Read the model definition and answer for the solid it produces. Units are mm, in the model's axes. Give positions to 0.01 mm unless a question says otherwise; leave off trailing zeros. Loops run counter-clockwise (first coordinate to the right, second up) from the corner with the lowest first, then second, coordinate; pieces in that order, holes last. Notation, with made-up numbers: (-36.5, 9.5) - (2.5, 9.5) arc R19 cw to (2.5, 27.5) - close; hole circle Ø5 at (34.5, -31). An arc over 180 degrees is marked (long way). Put each result on its own line as item: value. Start each with the question number.
1. Given pin 1 Ø1.5 at (y, z) = (30.5, 11) entering from -X; pin 2 Ø6 at (x, z) = (14, 3) entering from -Y; pin 3 Ø5 at (x, z) = (-12, 9.5) entering from +Y; pin 4 Ø1.5 at (x, z) = (-0.5, 7) entering from +Y, each flat-ended and moving along its own axis, determine where each tip first touches the part or whether it passes through.
2. A cutting plane is placed at D-D, the plane x = 11. Determine the outline of the cut face in (y, z), plus the area to 3 significant figures.
3. Consider L1, parallel to X at y = 7, z = 8; L2, parallel to Y at x = 0, z = 4.5; L3, parallel to Y at x = 11, z = 10.5. Determine where each line is inside the solid, lowest interval first. Write a range as from..to.
4. A cutting plane is placed at B-B, the plane z = 13.25. Determine the outline of the cut face in (x, y), plus the area to 3 significant figures.
5. A cutting plane is placed at C-C, the plane y = 27.3. Determine the outline of the cut face in (x, z), plus the area to 3 significant figures.
6. For a pull along X with two mould halves and no side action, classify faces 1 (the cylindrical face through (10.46, 3.76, 7.99)), 2 (the cylindrical face through (-16.57, -16.8, 7.76)), 3 (the cylindrical face through (-0.54, 24.86, 7.99)), 4 (the flat face through (0, 9, 0)) as released by +X, released by -X, zero draft, split by the parting line, or undercut.
7. A cutting plane is placed at A-A, the plane y = 6.2. Determine the outline of the cut face in (x, z), plus the area to 4 significant figures.
```python
from build123d import *

# Parameters (mm, degrees)
F1_DEPTH = 15.75
F2_R     = 2.5
F3_DEPTH = 15.751


with BuildPart() as f1:
    # F0 (on Top) → F1 (new body)
    with BuildSketch(Plane.XY):
        with BuildLine():
            ThreePointArc((-18, -13.3), (-16.535534, -16.835534), (-13, -18.3))
            Line((-13, -18.3), (13, -18.3))
            ThreePointArc((13, -18.3), (16.535534, -16.835534), (18, -13.3))
            Line((18, -13.3), (18, 18.3))
            ThreePointArc((18, 18.3), (0, 36.3), (-18, 18.3))
            Line((-18, 18.3), (-18, -13.3))
        make_face()
    extrude(amount=F1_DEPTH)

    # F2 (on face) → F3 (cut, through all)
    with BuildSketch(Plane.XY.offset(15.75)):
        with Locations((0, 27.3)):
            Circle(F2_R)
        with Locations((-11, 6.2)):
            Circle(F2_R)
        with Locations((11, 6.2)):
            Circle(F2_R)
    extrude(amount=-F3_DEPTH, mode=Mode.SUBTRACT)


solid = f1.part
```
Return value:
1. pin 1: stops at x = -13.89
1. pin 2: stops at y = -18.3
1. pin 3: stops at y = 33.59
1. pin 4: stops at y = 36.3
2. outline: (-18.3, 0) - (3.7, 0) - (3.7, 15.75) - (-18.3, 15.75) - close; (8.7, 0) - (32.55, 0) - (32.55, 15.75) - (8.7, 15.75) - close
2. area: 722 mm2
3. L1: x = -18..-13.37, -8.63..8.63, 13.37..18
3. L2: y = -18.3..24.8, 29.8..36.3
3. L3: y = -18.3..3.7, 8.7..32.55
4. outline: (-18, -13.3) arc R5 ccw to (-13, -18.3) - (13, -18.3) arc R5 ccw to (18, -13.3) - (18, 18.3) arc R18 ccw to (-18, 18.3) - close; hole circle Ø5 at (-11, 6.2); hole circle Ø5 at (0, 27.3); hole circle Ø5 at (11, 6.2)
4. area: 1,760 mm2
5. outline: (-15.59, 0) - (-2.5, 0) - (-2.5, 15.75) - (-15.59, 15.75) - close; (2.5, 0) - (15.59, 0) - (15.59, 15.75) - (2.5, 15.75) - close
5. area: 412 mm2
6. face 1: undercut
6. face 2: released by -X
6. face 3: undercut
6. face 4: zero draft
7. outline: (-18, 0) - (-13.5, 0) - (-13.5, 15.75) - (-18, 15.75) - close; (-8.5, 0) - (8.5, 0) - (8.5, 15.75) - (-8.5, 15.75) - close; (13.5, 0) - (18, 0) - (18, 15.75) - (13.5, 15.75) - close
7. area: 409.5 mm2
